Can you work these out from the model? Positions are in its coordinate system, mm. Give positions to 0.01 mm unless a question says otherwise; leave off trailing zeros. Order: outer loops, then holes, each group sorted by start corner. A loop starts at its lowest first (then second) coordinate and runs counter-clockwise, first axis right, second up. Notation, with made-up numbers: M 25,-3.75 L 71,-3.75 A10 ccw 71,14.25 Z; hole C 72,-18 d11. An arc over 180 degrees is marked long. Answer as a JSON object with one key per item and string values.
```python
from build123d import *

# Parameters (mm, degrees)
SKETCH_1_W              = 70
SKETCH_1_H              = 220
EXTRUDE_1_DEPTH         = 10
HOLE_WIZARD_M6_1_D      = 5
HOLE_WIZARD_18_0_18_1_D = 18
CHAMFER_1_SIZE          = 5


with BuildPart() as part:
    # 草圖1 → 伸長1 (new body)
    with BuildSketch(Plane(origin=(0, 0, 0), x_dir=(1, 0, 0), z_dir=(0, 1, 0))):
        Rectangle(SKETCH_1_W, SKETCH_1_H)
    extrude(amount=EXTRUDE_1_DEPTH)

    # M6 螺紋孔1 (through all)
    with Locations(Plane(origin=(0, 10, 0), x_dir=(-1, 0, 0), z_dir=(0, 1, 0))):
        with Locations((19, -59), (19, 59), (-5, -59), (-5, 59)):
            Hole(HOLE_WIZARD_M6_1_D / 2)

    # Ø18.0 (18) 直徑孔1 (through all)
    with Locations(Plane(origin=(0, 10, 0), x_dir=(-1, 0, 0), z_dir=(0, 1, 0))):
        with Locations((0, -90), (0, 90)):
            Hole(HOLE_WIZARD_18_0_18_1_D / 2)

    # 導角1
    chamfer_1_edges = [part.edges().sort_by_distance(p)[0] for p in [
        (-35, 5, -110),
        (35, 5, -110),
        (35, 5, 110),
        (-35, 5, 110),
    ]]
    chamfer(chamfer_1_edges, length=CHAMFER_1_SIZE)


solid = part.part
```
1) I want a section at C-C on y = 6.5. Write out the boundary of the cut face in (x, z).
Results found:
{"outline": "M -35,-105 L -30,-110 L 30,-110 L 35,-105 L 35,105 L 30,110 L -30,110 L -35,105 Z; hole C -19,-59 d5; hole C -19,59 d5; hole C 0,-90 d18; hole C 0,90 d18; hole C 5,-59 d5; hole C 5,59 d5"}
2) I need wall thicknesses on L1, parallel to X at y = 5.75, z = -59.5; L2, parallel to Z at x = 5, y = 6.5; L3, parallel to Z at x = -0.5, y = 4. Which ranges of each line are inside material? Lowest first, please.
Results found:
{"L1": "x = -35 to -21.45, -16.55 to 2.55, 7.45 to 35", "L2": "z = -110 to -97.48, -82.52 to -61.5, -56.5 to 56.5, 61.5 to 82.52, 97.48 to 110", "L3": "z = -110 to -98.99, -81.01 to 81.01, 98.99 to 110"}
3) I want a section at D-D on z = -90. Write out the boundary of the cut face in (x, y).
Results found:
{"outline": "M -35,0 L -9,0 L -9,10 L -35,10 Z; M 9,0 L 35,0 L 35,10 L 9,10 Z"}
4) I'm going to push a flat-ended pin straight in: pin 1 Ø8 at (x, z) = (-3.5, 8.5) entering from -Y. Where does the tip first touch, or does it pass through?
Results found:
{"pin 1": "stops at y = 0"}
5) I want a section at A-A on z = 59. Write out the boundary of the cut face in (x, y).
Results found:
{"outline": "M -35,0 L -21.5,0 L -21.5,10 L -35,10 Z; M -16.5,0 L 2.5,0 L 2.5,10 L -16.5,10 Z; M 7.5,0 L 35,0 L 35,10 L 7.5,10 Z"}
6) Thinking about a two-plate mould opening in X: for faces 1 (the face through (-1.951, 4.93, -98.786)), 2 (the face through (-32, 5, -108)), 3 (the face through (33, 5, 107)), which applies, pulls with the +X half, pulls with the -X half, needs draft (parallel to the pull), parting line crosses it, or undercut?
Results found:
{"face 1": "undercut", "face 2": "pulls with the -X half", "face 3": "pulls with the +X half"}
7) I want a section at B-B on x = -19. Write out the boundary of the cut face in (y, z).
Results found:
{"outline": "M 0,-110 L 10,-110 L 10,-61.5 L 0,-61.5 Z; M 0,-56.5 L 10,-56.5 L 10,56.5 L 0,56.5 Z; M 0,61.5 L 10,61.5 L 10,110 L 0,110 Z"}
